```python
from build123d import *

# Parameters (mm, degrees)
F0_R     = 35.566543
F2_R     = 15.24
F4_R     = 33.346959
F5_R     = 12.7
F7_R     = 9.525
F7_R_2   = 12.723879
F8_DEPTH = 12.7


with BuildPart() as f3:
    # F0 (on Top) → F3 section 0
    with BuildSketch(Plane.XY):
        Circle(F0_R)
    # F2 (on offset) → F3 section 1
    with BuildSketch(Plane.XY.offset(-50.8)):
        Circle(F2_R)
    loft()

    # F4 (on Top) → F6 section 0
    with BuildSketch(Plane.XY):
        Circle(F4_R)
    # F5 (on offset) → F6 section 1
    with BuildSketch(Plane.XY.offset(-50.8)):
        Circle(F5_R)
    loft(mode=Mode.SUBTRACT)

    # F7 (on offset) → F8 (join)
    with BuildSketch(Plane.XY.offset(-50.8)):
        with BuildLine():
            Line((-0.354267, -12.987269), (0, -12.987269))
            ThreePointArc((0, -12.987269), (12.987269, 0), (0, 12.987269))
            Line((0, 12.987269), (-0.354267, 12.987269))
            Line((-0.354267, 12.987269), (-41.074779, 12.987269))
            Line((-41.074779, 12.987269), (-41.074779, -12.987269))
            Line((-41.074779, -12.987269), (-0.354267, -12.987269))
        make_face()
        with Locations((-28.089361, 0)):
            Circle(F7_R, mode=Mode.SUBTRACT)
        Circle(F7_R_2, mode=Mode.SUBTRACT)
    extrude(amount=-F8_DEPTH)


solid = f3.part
```
Geometry check sheet. Reference: the model listing, model coordinates, mm. A direction names the side the tool comes from. Round coordinates to 2 decimals unless told otherwise and drop trailing zeros. Write each loop counter-clockwise with the first axis right and the second up, starting at its lowest first coordinate (ties: lowest second). Pieces come first, ordered by that corner, then holes. Notation, with made-up numbers: (34.25, 56) - (76.25, 56) arc R8 cw to (76.25, 61) - close; hole circle Ø10 at (-37.5, -33). An arc over 180 degrees is marked (long way). Write each question's results on one line, items separated by ' | '.
(1) Thickness scan on probe 1 along X at (y, z) = (1, -27); probe 2 along X at (y, z) = (-1.5, -28.5); probe 3 along Y at (x, z) = (10.5, -39.5). Record the ranges inside material, lowest first. Write a range as from..to.
Computed:
probe 1: x = -24.74..-22.35, 22.35..24.74 | probe 2: x = -24.12..-21.71, 21.71..24.12 | probe 3: y = -16.74..-13.74, 13.74..16.74
(2) Draft check along Z on faces 1 (the face through (19.634, 6.183, -31.4)), 2 (the face through (-20, 12.987, -57)), 3 (the face through (-17, 0, -50.8)), 4 (the face through (-20, 6, -63.5)). Enter one of: pulls with the +Z half, pulls with the -Z half, needs draft (parallel to the pull), parting line crosses it, or undercut.
Computed:
face 1: pulls with the +Z half | face 2: needs draft | face 3: undercut | face 4: pulls with the -Z half
(3) Set-up check for faces 5 (the face through (-21, -12.987, -57)), 6 (the face through (13, -2, -50.8)), 7 (the face through (-19.004, 2.861, -57.061)), 8 (the face through (10, 32, 0)), 9 (the face through (-41.075, 0, -57)): record each of +Z, -Z, +X, -X, +Y, -Y from which the full face is reachable in a straight line by a thin tool's end or side.
Computed:
face 5: -Z, +X, -X, -Y | face 6: -Z, +X | face 7: -Z | face 8: +Z, +X, -X, +Y, -Y | face 9: +Z, -Z, -X, +Y, -Y
(4) Sectioned sample at B-B, the plane z = -21.5. Enter the section's corners in (x, y).
Computed:
outline: circle Ø53.93 at (0, 0); hole circle Ø49.22 at (0, 0)
(5) Sectioned sample at A-A, the plane y = 0. Count the separate pieces of the cut face and the enclosed holes in it, plus the area to 3 significant figures.
Computed:
separate pieces: 3 | enclosed holes: 0 | area: 363 mm^2
(6) Depth check by flat-ended pin: pin 1 Ø8 at (x, y) = (-25, -4.5) entering from -Z; pin 2 Ø14 at (x, z) = (-15, -57.5) entering from -Y; pin 3 Ø12 at (x, y) = (-29, 5) entering from +Z; pin 4 Ø12 at (x, z) = (14.5, -50.5) entering from +Y. Enter the tip coordinate at first touch or a pass-through.
Computed:
pin 1: stops at z = -35.4 | pin 2: stops at y = -12.99 | pin 3: stops at z = 0 | pin 4: stops at y = 13.72
